```python
from build123d import *

# Parameters (mm, degrees)
SKETCH1_R           = 6.5
BOSS_EXTRUDE1_DEPTH = 11
BOSS_EXTRUDE2_DEPTH = 48
SKETCH2_R           = 12
CUT_EXTRUDE1_DEPTH  = 135.648061082


with BuildPart() as part:
    # Sketch1 → Boss-Extrude1 (new body)
    with BuildSketch(Plane.XY):
        with BuildLine():
            Line((15, 0), (15, 54))
            ThreePointArc((15, 54), (17.928932188, 61.071067812), (25, 64))
            Line((25, 64), (-25, 64))
            ThreePointArc((-25, 64), (-17.928932188, 61.071067812), (-15, 54))
            Line((-15, 54), (-15, 0))
            ThreePointArc((-15, 0), (0, -15), (15, 0))
        make_face()
        Circle(SKETCH1_R, mode=Mode.SUBTRACT)
        with Locations((0, 30)):
            Circle(SKETCH1_R, mode=Mode.SUBTRACT)
    extrude(amount=-BOSS_EXTRUDE1_DEPTH)

    # Sketch1_3 → Boss-Extrude2 (add)
    with BuildSketch(Plane.XY):
        Polygon((27.810759955, 82), (0, 82), (0, 64), (25, 64), (38.810759955, 64), (38.810759955, 99), (27.810759955, 99), align=None)
        Polygon((0, 64), (0, 82), (-27.810759955, 82), (-27.810759955, 99), (-38.810759955, 99), (-38.810759955, 64), (-25, 64), align=None)
    extrude(amount=-BOSS_EXTRUDE2_DEPTH)

    # Sketch2 → Cut-Extrude1 (cut, through all)
    with BuildSketch(Plane(origin=(38.810759955, 0, 0), x_dir=(0, 0, -1), z_dir=(1, 0, 0))):
        with Locations((24, 99)):
            Circle(SKETCH2_R)
    extrude(amount=-CUT_EXTRUDE1_DEPTH, mode=Mode.SUBTRACT)


solid = part.part
```
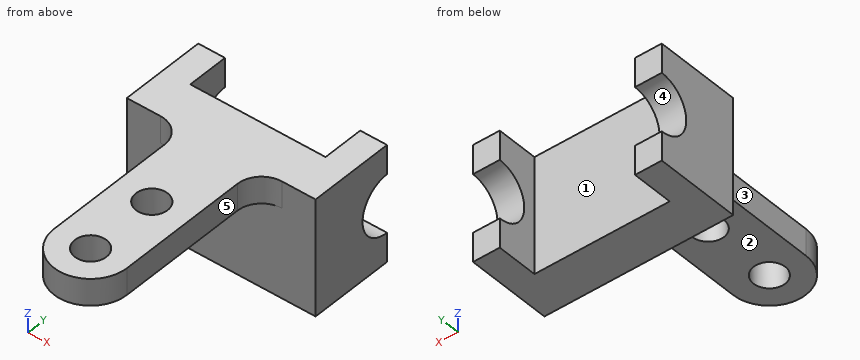
Verification items for the finished model (mm, model axes). Face numbers are marked on the shaded views. A direction names the side the tool comes from. Round coordinates to 2 decimals unless told otherwise and drop trailing zeros. Write each loop counter-clockwise with the first axis right and the second up, starting at its lowest first coordinate (ties: lowest second). Pieces come first, ordered by that corner, then holes. Notation, with made-up numbers: (-37, 84.25) - (-2, 84.25) arc R15 ccw to (-2, 90.25) - close; hole circle Ø2 at (2.5, -7.75). An arc over 180 degrees is marked (long way). Answer as a JSON object with one key per item and string values. Group by question number.
Q1. Tool access check on the marked faces 4 and 5. Record the directions out of +Z, -Z, +X, -X, +Y, -Y that give a thin tool (end or side, any length) a straight path to the whole face; none if there is none.
Q2. Section check B-B, the plane x = 0. Enter the section's corners in (y, z).
Q3. Thickness scan on line 1 (Y direction, x = 0, z = -3.5); line 2 (Z direction, x = -3, y = 62.5); line 3 (X direction, y = 17.5, z = -4.5). Record the ranges inside material, lowest first.
Q4. Section check C-C, the plane z = -4. Enter the section's corners in (x, y).
Q5. Section check D-D, the plane z = -39.5. Enter the section's corners in (x, y).
Q6. Mould release check, pull along X, two halves, no side actions. Record for the marked faces 1, 2 and 3: released by +X, released by -X, zero draft, split by the parting line, or undercut.
Q7. Go/stop test with flat-tipped pins: pin 1 Ø14.5 at (x, z) = (0.5, -34) entering from +Y; pin 2 Ø12 at (y, z) = (15.5, -6) entering from +X; pin 3 Ø8 at (x, y) = (0, 0) entering from -Z; pin 4 Ø12 at (y, z) = (35, -4) entering from -X. Record where each tip stops, or that it passes through.
Q8. Section check A-A, the plane y = 30. Enter the section's corners in (x, z), plus the area to 3 significant figures.
Found:
{
 "1": {"face 4": "+X, -X, +Y", "face 5": "+Z, -Z, +X, -Y"},
 "2": {"outline": "(-15, -11) - (-6.5, -11) - (-6.5, 0) - (-15, 0) - close; (6.5, -11) - (23.5, -11) - (23.5, 0) - (6.5, 0) - close; (36.5, -11) - (64, -11) - (64, -48) - (82, -48) - (82, 0) - (36.5, 0) - close"},
 "3": {"line 1": "y = -15 to -6.5, 6.5 to 23.5, 36.5 to 82", "line 2": "z = -11 to 0", "line 3": "x = -15 to 15"},
 "4": {"outline": "(-38.81, 64) - (-25, 64) arc R10 cw to (-15, 54) - (-15, 0) arc R15 ccw to (15, 0) - (15, 54) arc R10 cw to (25, 64) - (38.81, 64) - (38.81, 99) - (27.81, 99) - (27.81, 82) - (-27.81, 82) - (-27.81, 99) - (-38.81, 99) - close; hole circle Ø13 at (0, 0); hole circle Ø13 at (0, 30)"},
 "5": {"outline": "(-38.81, 64) - (38.81, 64) - (38.81, 99) - (27.81, 99) - (27.81, 82) - (-27.81, 82) - (-27.81, 99) - (-38.81, 99) - close"},
 "6": {"face 1": "undercut", "face 2": "zero draft", "face 3": "released by -X"},
 "7": {"pin 1": "stops at y = 82", "pin 2": "stops at x = 15", "pin 3": "passes through", "pin 4": "stops at x = -15"},
 "8": {"outline": "(-15, -11) - (-6.5, -11) - (-6.5, 0) - (-15, 0) - close; (6.5, -11) - (15, -11) - (15, 0) - (6.5, 0) - close", "area": "187 mm^2"}
}
